Source: CAD feature listing. Evaluate the final solid. Frame: model axes, mm. A direction names the side the tool comes from. Round coordinates to 2 decimals unless told otherwise and drop trailing zeros. Order: outer loops, then holes, each group sorted by start corner. A loop starts at its lowest first (then second) coordinate and runs counter-clockwise, first axis right, second up. Notation, with made-up numbers: (42, 49.5) -> (73, 49.5) arc R20 cw to (73, 84.5) -> close; hole circle Ø10 at (57, 52.5). An arc over 180 degrees is marked (long way). One line per item, written item: value. Start each with the question number.
1) Reachability of faces 4 (the face through (22, 13, 14)), 5 (the face through (-29, 0, 0)), 6 (the face through (-18, -13, -14)) from +Z, -Z, +X, -X, +Y, -Y: full face, straight path, thin tool, end or side. Return the list, or none.
2) Section B-B (y = -4.5). Return the cut outline in (x, z).
3) Pin query (flat end, axial travel): P1, Ø1.2, axis at x = -19.5, z = -14, coming from the -Y side; P2, Ø6.5, axis at x = 18, z = 14, coming from the -Y side; P3, Ø4, axis at x = -19, z = -13.5, coming from the +Y side. Return the tip coordinate at first contact, or that it passes through.
4) Section D-D (y = 2). Return the cut outline in (x, z), and give its area (3 significant figures).
5) Mould query, pull axis X, two halves, no side actions, for faces 1 (the face through (-13, 18, 2)), 2 (the face through (22.7, 14.49, -16.95)), 3 (the face through (28.287, 0.189, -19.248)). Classes: pulls with the +X half, pulls with the -X half, needs draft (parallel to the pull), parting line crosses it, or undercut.
6) Section A-A (z = 0). Return the cut outline in (x, y), and give its area (3 significant figures).
7) Ray query, L1, parallel to X at y = 10, z = 14; L2, parallel to Y at x = -20, z = -6.5; L3, parallel to Y at x = 83, z = 13. Return the intervals inside material, ascending.
8) Section C-C (x = 6). Return the cut outline in (y, z), and give its area (3 significant figures).
```python
from build123d import *

# Parameters (mm, degrees)
BOSS_EXTRUDE1_DEPTH = 13.5
SKETCH2_R           = 4
BOSS_EXTRUDE2_DEPTH = 2
SKETCH3_R           = 2
CUT_EXTRUDE1_DEPTH  = 6
SKETCH6_R           = 9.5
BOSS_EXTRUDE5_DEPTH = 4.5
SKETCH4_R           = 4
BOSS_EXTRUDE3_DEPTH = 15
SKETCH5_R           = 15.5
BOSS_EXTRUDE4_DEPTH = 62
SKETCH7_R           = 4
CUT_EXTRUDE2_DEPTH  = 1.7


with BuildPart() as part:
    # Sketch1 → Boss-Extrude1 (new, symmetric)
    with BuildSketch(Plane(origin=(0, 0, 0), x_dir=(1, 0, 0), z_dir=(0, 1, 0))):
        with BuildLine():
            Line((-26.5, -20), (26.5, -20))
            ThreePointArc((26.5, -20), (28.267766953, -19.267766953), (29, -17.5))
            Line((29, -17.5), (29, 17.5))
            ThreePointArc((29, 17.5), (28.267766953, 19.267766953), (26.5, 20))
            Line((26.5, 20), (-26.5, 20))
            ThreePointArc((-26.5, 20), (-28.267766953, 19.267766953), (-29, 17.5))
            Line((-29, 17.5), (-29, -17.5))
            ThreePointArc((-29, -17.5), (-28.267766953, -19.267766953), (-26.5, -20))
        make_face()
    extrude(amount=BOSS_EXTRUDE1_DEPTH, both=True)

    # Sketch2 → Boss-Extrude2 (add)
    with BuildSketch(Plane(origin=(0, 13.5, 0), x_dir=(1, 0, 0), z_dir=(0, 1, 0))):
        with Locations(Location((-20, 14, 0), (0, 0, 270))):
            Circle(SKETCH2_R)
        with Locations(Location((-20, -14, 0), (0, 0, 270))):
            Circle(SKETCH2_R)
        with Locations(Location((20, -14, 0), (0, 0, 270))):
            Circle(SKETCH2_R)
        with Locations(Location((20, 14, 0), (0, 0, 270))):
            Circle(SKETCH2_R)
    boss_extrude2 = extrude(amount=BOSS_EXTRUDE2_DEPTH)

    # Sketch3 → Cut-Extrude1 (cut)
    with BuildSketch(Plane(origin=(0, 15.5, 0), x_dir=(1, 0, 0), z_dir=(0, 1, 0))):
        with Locations(Location((-20, 14, 0), (0, 0, 270))):
            Circle(SKETCH3_R)
        with Locations(Location((20, 14, 0), (0, 0, 270))):
            Circle(SKETCH3_R)
        with Locations(Location((20, -14, 0), (0, 0, 270))):
            Circle(SKETCH3_R)
        with Locations(Location((-20, -14, 0), (0, 0, 270))):
            Circle(SKETCH3_R)
    cut_extrude1 = extrude(amount=-CUT_EXTRUDE1_DEPTH, mode=Mode.SUBTRACT)

    # Sketch6 → Boss-Extrude5 (add)
    with BuildSketch(Plane(origin=(0, 13.5, 0), x_dir=(1, 0, 0), z_dir=(0, 1, 0))):
        with Locations(Location((-9, 0, 0), (0, 0, 270))):
            Circle(SKETCH6_R)
    boss_extrude5 = extrude(amount=BOSS_EXTRUDE5_DEPTH)

    # Sketch4 → Boss-Extrude3 (add)
    with BuildSketch(Plane(origin=(0, 18, 0), x_dir=(1, 0, 0), z_dir=(0, 1, 0))):
        with Locations(Location((-9, 0, 0), (0, 0, 270))):
            Circle(SKETCH4_R)
    extrude(amount=BOSS_EXTRUDE3_DEPTH)

    # Sketch5 → Boss-Extrude4 (add)
    with BuildSketch(Plane(origin=(29, 0, 0), x_dir=(0, 0, -1), z_dir=(1, 0, 0))):
        with Locations(Location((0, -4.5, 0), (0, 0, 215.49593265))):
            Circle(SKETCH5_R)
    extrude(amount=BOSS_EXTRUDE4_DEPTH)

    # Mirror2: Boss-Extrude2, Cut-Extrude1, Boss-Extrude5 across plane
    add(boss_extrude2.mirror(Plane.ZX))
    add(cut_extrude1.mirror(Plane.ZX), mode=Mode.SUBTRACT)
    add(boss_extrude5.mirror(Plane.ZX))

    # Sketch7 → Cut-Extrude2 (cut)
    with BuildSketch(Plane.XZ.offset(18)):
        with Locations(Location((-9, 0, 0), (0, 0, 90))):
            Circle(SKETCH7_R)
    extrude(amount=-CUT_EXTRUDE2_DEPTH, mode=Mode.SUBTRACT)


solid = part.part
```
Findings:
1. face 4: +Y
1. face 5: +Z, -Z, -X, +Y, -Y
1. face 6: -Y
2. outline: (-29, -17.5) arc R2.5 ccw to (-26.5, -20) -> (26.5, -20) arc R2.5 ccw to (29, -17.5) -> (29, -15.5) -> (91, -15.5) -> (91, 15.5) -> (29, 15.5) -> (29, 17.5) arc R2.5 ccw to (26.5, 20) -> (-26.5, 20) arc R2.5 ccw to (-29, 17.5) -> close
3. P1: y = -9.5
3. P2: y = -15.5
3. P3: y = 15.5
4. outline: (-29, -17.5) arc R2.5 ccw to (-26.5, -20) -> (26.5, -20) arc R2.5 ccw to (29, -17.5) -> (29, -14.07) -> (91, -14.07) -> (91, 14.07) -> (29, 14.07) -> (29, 17.5) arc R2.5 ccw to (26.5, 20) -> (-26.5, 20) arc R2.5 ccw to (-29, 17.5) -> close
4. area: 4,060 mm2
5. face 1: needs draft
5. face 2: undercut
5. face 3: pulls with the +X half
6. outline: (-29, -13.5) -> (-18.5, -13.5) -> (-18.5, -18) -> (-13, -18) -> (-13, -16.3) -> (-5, -16.3) -> (-5, -18) -> (0.5, -18) -> (0.5, -13.5) -> (29, -13.5) -> (29, -20) -> (91, -20) -> (91, 11) -> (29, 11) -> (29, 13.5) -> (0.5, 13.5) -> (0.5, 18) -> (-5, 18) -> (-5, 33) -> (-13, 33) -> (-13, 18) -> (-18.5, 18) -> (-18.5, 13.5) -> (-29, 13.5) -> close
6. area: 3,770 mm2
7. L1: -29 to -22, -18 to 18, 22 to 29
7. L2: -13.5 to 13.5
7. L3: -12.94 to 3.94
8. outline: (-13.5, -20) -> (13.5, -20) -> (13.5, 20) -> (-13.5, 20) -> close
8. area: 1,080 mm2
